from build123d import *

# Parameters (mm, degrees)
BOSS_EXTRUDE1_DEPTH     = 20
CUT_EXTRUDE1_DEPTH      = 1
CUT_EXTRUDE1_DEPTH_BACK = 21
SKETCH4_R               = 2.6
CUT_EXTRUDE2_DEPTH      = 6
SKETCH5_R               = 2.6
CUT_EXTRUDE3_DEPTH      = 6


with BuildPart() as part:
    # Sketch1 → Boss-Extrude1 (new body)
    with BuildSketch(Plane.XY):
        Polygon((0, 0), (0, 50), (50, 0), align=None)
    extrude(amount=BOSS_EXTRUDE1_DEPTH)

    # Sketch2 → Cut-Extrude1 (cut, two sides)
    with BuildSketch(Plane.XY.offset(20)) as cut_extrude1_sk:
        Polygon((5, 182.279220614), (5, 45), (5, 5), (45, 5), (182.279220614, 5), (376.421356237, 199.142135624), (199.142135624, 376.421356237), align=None)
    extrude(amount=CUT_EXTRUDE1_DEPTH, mode=Mode.SUBTRACT)
    extrude(cut_extrude1_sk.sketch, amount=-CUT_EXTRUDE1_DEPTH_BACK, mode=Mode.SUBTRACT)

    # Sketch4 → Cut-Extrude2 (cut, through all)
    with BuildSketch(Plane(origin=(5, 0, 0), x_dir=(0, 0, -1), z_dir=(1, 0, 0))):
        with Locations((-10, 35)):
            Circle(SKETCH4_R)
        with Locations((-10, 25)):
            Circle(SKETCH4_R)
        with Locations((-10, 15)):
            Circle(SKETCH4_R)
    extrude(amount=-CUT_EXTRUDE2_DEPTH, mode=Mode.SUBTRACT)

    # Sketch5 → Cut-Extrude3 (cut, through all)
    with BuildSketch(Plane(origin=(0, 5, 0), x_dir=(1, 0, 0), z_dir=(0, 1, 0))):
        with Locations((35, -10)):
            Circle(SKETCH5_R)
        with Locations((25, -10)):
            Circle(SKETCH5_R)
        with Locations((15, -10)):
            Circle(SKETCH5_R)
    extrude(amount=-CUT_EXTRUDE3_DEPTH, mode=Mode.SUBTRACT)


solid = part.part
Check sheet for the modelled part. Datum: model origin and axes. Units: mm. A direction names the side the tool comes from. Round coordinates to 2 decimals unless told otherwise and drop trailing zeros. Loops run counter-clockwise (first coordinate to the right, second up) from the corner with the lowest first, then second, coordinate; pieces in that order, holes last. Notation, with made-up numbers: (-11, -9) - (16, -9) arc R28 ccw to (16, 29) - close; hole circle Ø3 at (11.5, -28.75). An arc over 180 degrees is marked (long way). Answer as CSV lines item,"result". Start each with the question number.
Item 1: Section check B-B (y = 35). Record the boundary of the cut face in (x, z).
Item 2: Scan lines: line 1 (Z direction, x = 15, y = 1); line 2 (Y direction, x = 9.5, z = 13.25). Record each from-to range of solid material in increasing order. Write a range as [from, to].
Item 3: Release check for a two-part mould opening along Y. For faces 1 (the flat face through (0, 25, 5)), 2 (the flat face through (2, 48, 10)), 3 (the cylindrical face through (2.535, 27.578, 10.338)) record: +Y half, -Y half, draft (parallel to the pull), parting line (faces both ways), or undercut.
Item 4: Depth check by flat-ended pin: P1, Ø5, axis at x = 24.5, z = 6, coming from the -Y side; P2, Ø10, axis at x = 38, z = 10, coming from the +Y side; P3, Ø1.5, axis at y = 39, z = 14.5, coming from the +X side. Enter the tip coordinate at first touch or a pass-through.
Item 5: Section check D-D (z = 14). Record the boundary of the cut face in (x, y).
Item 6: Set-up check for faces 4 (the flat face through (5, 21, 10)), 5 (the cylindrical face through (17.4, 2.5, 11)): record each of +Z, -Z, +X, -X, +Y, -Y from which the full face is reachable in a straight line by a thin tool's end or side.
Item 7: Section check A-A (z = 9). Count the separate pieces of the cut face and the enclosed holes in it, and give its area (3 significant figures).
Report:
1,outline,"(0, 0) - (5, 0) - (5, 7.4) - (0, 7.4) - close; (0, 12.6) - (5, 12.6) - (5, 20) - (0, 20) - close"
2,line 1,"z = [0, 7.4], [12.6, 20]"
2,line 2,"y = [0, 5]"
3,face 1,"draft"
3,face 2,"+Y half"
3,face 3,"undercut"
4,P1,"stops at y = 0"
4,P2,"stops at y = 5"
4,P3,"stops at x = 5"
5,outline,"(0, 0) - (50, 0) - (45, 5) - (5, 5) - (5, 45) - (0, 50) - close"
6,face 4,"+Z, -Z, +X, +Y"
6,face 5,"+Y, -Y"
7,separate pieces,"7"
7,enclosed holes,"0"
7,area,"306 mm2"
